Print and shaded views of the part. All mm, measured from the part's lowest x, y and z. A direction names the side the tool comes from. Give positions to 0.01 mm unless a question says otherwise; leave off trailing zeros. Loops run counter-clockwise (first coordinate to the right, second up) from the corner with the lowest first, then second, coordinate; pieces in that order, holes last. Notation, with made-up numbers: M -33,42.5 L -27,42.5 A24 ccw -27,76.5 Z; hole C -30,71.5 d10. An arc over 180 degrees is marked long. Put each result on its own line as item: value. Start each with the question number.
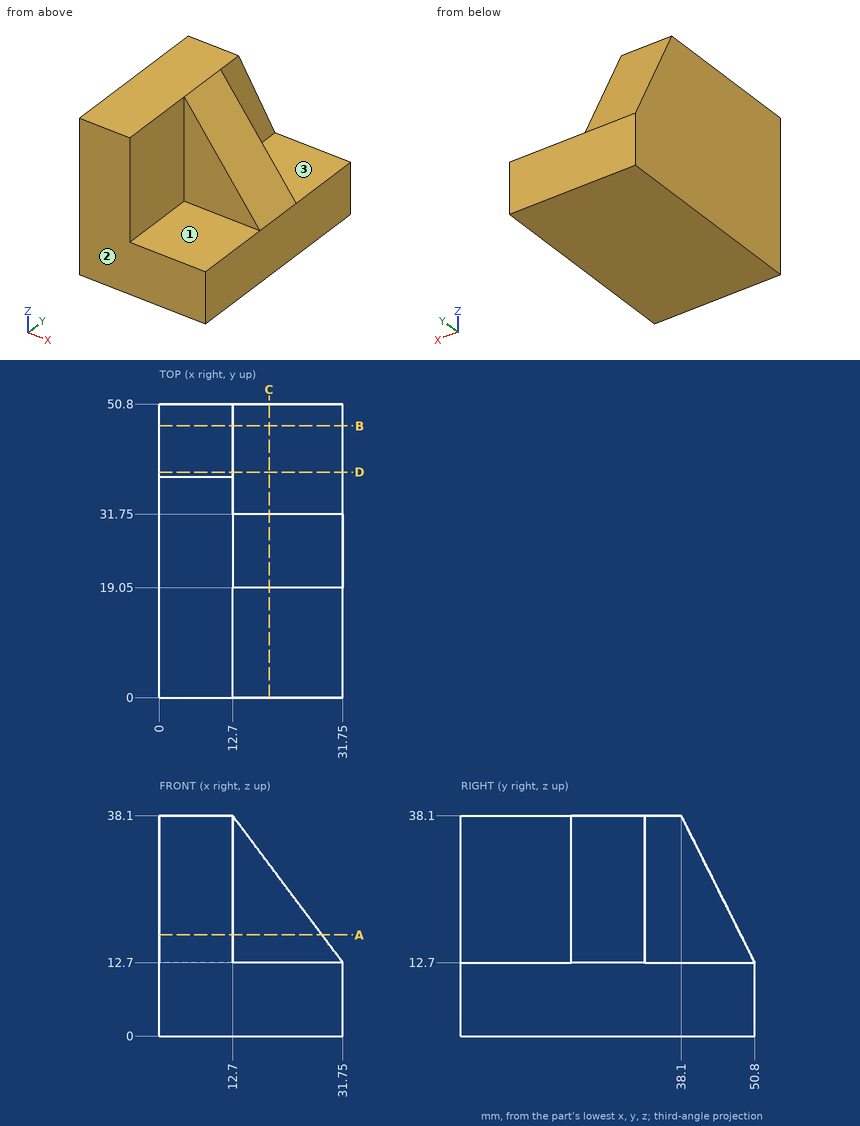
1) Which spindle directions (+Z, -Z, +X, -X, +Y, -Y) get a long thin tool onto all of the face, cutting with end or side? Do the marked faces 1, 2 and 3. Say none if no direction does.
2) Band-saw the part on A-A on z = 17.5. Give the cut face in (x, y).
3) Band-saw the part on B-B on y = 47. Give the cut face in (x, z), then the cut area to 3 significant figures.
4) Wall check: L1, parallel to X at y = 11.5, z = 24; L2, parallel to Y at x = 22, z = 17.5. Give the ranges that are in metal, low to high.
5) Pin check, flat tips, straight feed: pin 1 Ø4 at (x, y) = (12, 43) entering from +Z; pin 2 Ø5.5 at (x, z) = (23.5, 23) entering from -Y; pin 3 Ø6 at (y, z) = (10.5, 34) entering from -X; pin 4 Ø5.5 at (y, z) = (13, 25) entering from +X. Stop position of each tip, or through.
6) Band-saw the part on C-C on x = 19. Give the cut face in (y, z), then the cut area to 3 significant figures.
7) Band-saw the part on D-D on y = 39. Give the cut face in (x, z).
Evaluation:
1. face 1: +Z, +X, -Y
1. face 2: +Z, -Z, +X, -X, -Y
1. face 3: +Z, +X, +Y
2. outline: M 0,0 L 12.7,0 L 12.7,19.05 L 28.15,19.05 L 28.15,31.75 L 12.7,31.75 L 12.7,48.4 L 0,48.4 Z
3. outline: M 0,0 L 31.75,0 L 31.75,12.7 L 12.7,12.7 L 12.7,20.3 L 0,20.3 Z
3. area: 500 mm2
4. L1: 0 to 12.7
4. L2: 19.05 to 31.75
5. pin 1: z = 32.3
5. pin 2: y = 19.05
5. pin 3: x = 0
5. pin 4: x = 12.7
6. outline: M 0,0 L 50.8,0 L 50.8,12.7 L 31.75,12.7 L 31.75,29.7 L 19.05,29.7 L 19.05,12.7 L 0,12.7 Z
6. area: 861 mm2
7. outline: M 0,0 L 31.75,0 L 31.75,12.7 L 12.7,12.7 L 12.7,36.3 L 0,36.3 Z
